Design review of the part built by this model. Coordinates are the model's own, in mm. Face numbers are marked on the shaded views. A direction names the side the tool comes from. Give positions to 0.01 mm unless a question says otherwise; leave off trailing zeros. Loops run counter-clockwise (first coordinate to the right, second up) from the corner with the lowest first, then second, coordinate; pieces in that order, holes last. Notation, with made-up numbers: M 86.25,-5.5 L 94.25,-5.5 A20 cw 94.25,6.5 Z; hole C -6,73 d10. An arc over 180 degrees is marked long. Use a Markdown table: item, result. Add a question column.
(1) For probe 1 along Y at (x, z) = (-2, -5.5); probe 2 along X at (y, z) = (-12, -2.5); probe 3 along Y at (x, z) = (13.5, -8.25), list the stretches that pass through material, from the lowest coordinate up.
(2) Add section D-D, the plane z = -4.75. State how many separate pieces and enclosed holes the cut face has, then the cut area to 3 significant figures.
(3) Insertion check: pin 1 Ø16 at (x, y) = (-22.52, -13) entering from -Z; pin 2 Ø3 at (x, z) = (38, -3.5) entering from +Y; pin 3 Ø5 at (y, z) = (-33.5, -9) entering from +X; pin 4 Ø4 at (x, z) = (19, -8.5) entering from +Y. Each pin has a flat end and moves straight along its axis. Give the tip position at first contact, or say it passes through.
(4) For the marked faces 4 and 5, list the 3-axis set-ups (+Z, -Z, +X, -X, +Y, -Y) from which the entire face can be reached by the end or side of a thin tool; tool diameter is ignored.
(5) Add section A-A, the plane x = 0. Give the boundary of the cut face in (y, z), then the cut area to 3 significant figures.
(6) Draft analysis for pull direction X (two halves, no side actions). For the marked faces 1, 2 and 3, state which applies: pulls with the +X half, pulls with the -X half, needs draft (parallel to the pull), parting line crosses it, or undercut.
(7) Add section C-C, the plane y = -35. Give the boundary of the cut face in (x, z).
(8) Add section B-B, the plane y = 0. Give the boundary of the cut face in (x, z).
```python
from build123d import *

# Parameters (mm, degrees)
SKETCH2_R           = 5
SKETCH2_R_2         = 18
BOSS_EXTRUDE1_DEPTH = 10


with BuildPart() as part:
    # Sketch2 → Boss-Extrude1 (new body)
    with BuildSketch(Plane.XY):
        with BuildLine():
            ThreePointArc((29.444863729, -17), (0, 34), (-29.444863729, -17))
            ThreePointArc((-29.444863729, -17), (-30.432675575, -26.289059694), (-38.97114317, -22.5))
            ThreePointArc((-38.97114317, -22.5), (-49.216333699, -19.754809472), (-51.961524227, -30))
            ThreePointArc((-51.961524227, -30), (0, -60), (51.961524227, -30))
            ThreePointArc((51.961524227, -30), (49.216333699, -19.754809472), (38.97114317, -22.5))
            ThreePointArc((38.97114317, -22.5), (30.429409054, -26.294717474), (29.444863729, -17))
        make_face()
        with Locations((22.516660498, -13)):
            Circle(SKETCH2_R, mode=Mode.SUBTRACT)
        with Locations((0, -26)):
            Circle(SKETCH2_R, mode=Mode.SUBTRACT)
        with Locations((-22.516660498, -13)):
            Circle(SKETCH2_R, mode=Mode.SUBTRACT)
        with Locations((-22.516660498, 13)):
            Circle(SKETCH2_R, mode=Mode.SUBTRACT)
        with Locations((0, 26)):
            Circle(SKETCH2_R, mode=Mode.SUBTRACT)
        with Locations((22.516660498, 13)):
            Circle(SKETCH2_R, mode=Mode.SUBTRACT)
        with BuildLine():
            ThreePointArc((-49.903995186, -28.812085055), (-48.028418753, -21.812338512), (-41.028672211, -23.687914945))
            ThreePointArc((-41.028672211, -23.687914945), (0, -48.031541814), (41.028672211, -23.687914945))
            ThreePointArc((41.028672211, -23.687914945), (48.028418753, -21.812338512), (49.903995186, -28.812085055))
            ThreePointArc((49.903995186, -28.812085055), (0, -57.624170109), (-49.903995186, -28.812085055))
        make_face(mode=Mode.SUBTRACT)
        Circle(SKETCH2_R_2, mode=Mode.SUBTRACT)
    extrude(amount=-BOSS_EXTRUDE1_DEPTH)


solid = part.part
```
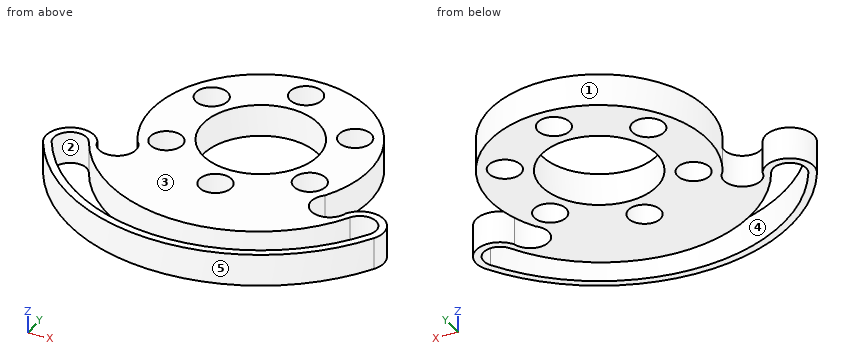
Established:
| question | item | result |
|---|---|---|
| 1 | probe 1 | -59.97 to -57.59, -47.99 to -30.58, -21.42 to -17.89, 17.89 to 21.42, 30.58 to 33.94 |
| 1 | probe 2 | -31.81 to -27.42, -17.62 to -13.42, 13.42 to 17.62, 27.42 to 31.81 |
| 1 | probe 3 | -58.46 to -56.02, -46.04 to -11.91, 11.91 to 31.2 |
| 2 | separate pieces | 1 |
| 2 | enclosed holes | 8 |
| 2 | area | 3,570 mm^2 |
| 3 | pin 1 | z = -10 |
| 3 | pin 2 | y = -21.71 |
| 3 | pin 3 | x = 51.37 |
| 3 | pin 4 | y = 29.44 |
| 4 | face 4 | +Z, -Z |
| 4 | face 5 | +Z, -Z, -Y |
| 5 | outline | M -60,-10 L -57.62,-10 L -57.62,0 L -60,0 Z; M -48.03,-10 L -31,-10 L -31,0 L -48.03,0 Z; M -21,-10 L -18,-10 L -18,0 L -21,0 Z; M 18,-10 L 21,-10 L 21,0 L 18,0 Z; M 31,-10 L 34,-10 L 34,0 L 31,0 Z |
| 5 | area | 284 mm^2 |
| 6 | face 1 | parting line crosses it |
| 6 | face 2 | undercut |
| 6 | face 3 | needs draft |
| 7 | outline | M -48.73,-10 L -45.78,-10 L -45.78,0 L -48.73,0 Z; M -32.38,-10 L 32.38,-10 L 32.38,0 L -32.38,0 Z; M 45.78,-10 L 48.73,-10 L 48.73,0 L 45.78,0 Z |
| 8 | outline | M -34,-10 L -18,-10 L -18,0 L -34,0 Z; M 18,-10 L 34,-10 L 34,0 L 18,0 Z |
